The listing builds one solid part. Answer for the finished solid, in the listing's coordinates (mm). Face numbers are marked on the shaded views. A direction names the side the tool comes from. Round coordinates to 2 decimals unless told otherwise and drop trailing zeros. Order: outer loops, then holes, each group sorted by start corner. A loop starts at its lowest first (then second) coordinate and runs counter-clockwise, first axis right, second up. Notation, with made-up numbers: (66.25, 55) - (123.25, 55) arc R29 ccw to (123.25, 84) - close; hole circle Ø8 at (-2, 18.5). An arc over 180 degrees is marked (long way). Use CSV: the item, a comma, the result in double quotes. Start each with the question number.
Item 1: Find section D-D, the plane y = -2.1. Give the vertices of the cut face in (x, z), plus the area to 3 significant figures.
Item 2: For the marked faces 1 and 2, determine the directions among +Z, -Z, +X, -X, +Y, -Y from which every point of the face is accessible in a straight line to the end or side of a thin tool.
Item 3: Straight lines are drawn through the part: line 1 along Z through (x, y) = (-2.35, -1); line 2 along Z through (x, y) = (2.45, 0.4); line 3 along Y through (x, z) = (0, 1.5). For each, find the intervals that lie inside material, in ascending order. Write a range as [from, to].
Item 4: Flat-ended cylindrical pins translate along their axes: P1, Ø0.5, axis at x = 0, y = 0, coming from the +Z side; P2, Ø3, axis at x = 1, z = 23, coming from the +Y side; P3, Ø1.5, axis at x = -2, y = 0, coming from the -Z side; P4, Ø1.3, axis at x = -0.5, z = 26.5, coming from the -Y side. Find the tip coordinate at first contact, or state that the pin passes through.
Item 5: Find section A-A, the plane x = 0. Give the vertices of the cut face in (y, z).
Item 6: Find section C-C, the plane z = 18. Give the vertices of the cut face in (x, y).
Item 7: Find section B-B, the plane y = 0. Give the vertices of the cut face in (x, z).
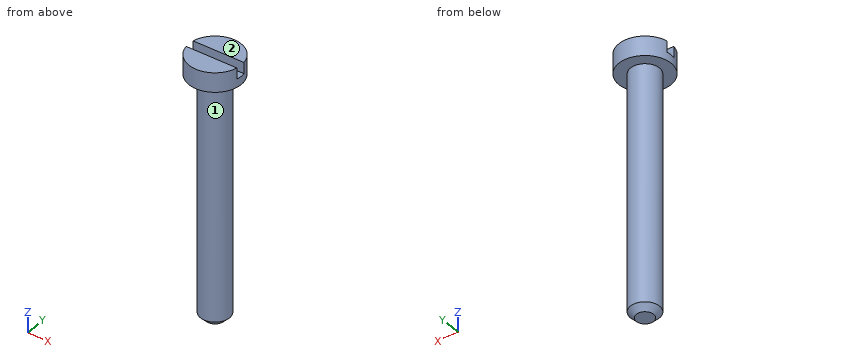
Solid Edge part; units mm, degrees
sketch "Sketch1" plane through (0, 0, 0) normal (0, 0, 1) x (1, 0, 0)
  circle A0 centre (0, 0) radius 1.5
extrude "Protrusion1" add sketch "Sketch1" along normal blind 25
chamfer "Chaflán_1" distance 0.6 angle 45 1 edges at (-1.5, 0, 0)
sketch "Sketch2" plane through (0, 0, 25) normal (0, 0, 1) x (1, 0, 0)
  circle A0 centre (0, 0) radius 2.7
extrude "ProtrusiónExtruida_3" add sketch "Sketch2" along normal blind 2
sketch "Sketch3" plane through (0, 0, 27) normal (0, 0, 1) x (0, 1, 0)
  line L0 (0.5, -3.2084) -> (-0.5, -3.2084)
  line L1 (-0.5, -3.2084) -> (-0.5, 3.2084)
  line L2 (-0.5, 3.2084) -> (0.5, 3.2084)
  line L3 (0.5, 3.2084) -> (0.5, -3.2084)
extrude "VaciadoExtruido_5" cut sketch "Sketch3" against normal blind 1.148
properties material "Acero inoxidable, 303"
Worked out:
1,outline,"(-1.7, 25) - (1.7, 25) - (1.7, 27) - (-1.7, 27) - close"
1,area,"6.79 mm²"
2,face 1,"-Z"
2,face 2,"+Z, +X, -X, +Y, -Y"
3,line 1,"z = [25, 27]"
3,line 2,"z = [25, 25.85]"
3,line 3,"y = [-1.5, 1.5]"
4,P1,"stops at z = 25.85"
4,P2,"stops at y = 1.5"
4,P3,"stops at z = 0.35"
4,P4,"stops at y = -2.7"
5,outline,"(-2.7, 25) - (-1.5, 25) - (-1.5, 0.6) - (-0.9, 0) - (0.9, 0) - (1.5, 0.6) - (1.5, 25) - (2.7, 25) - (2.7, 27) - (0.5, 27) - (0.5, 25.85) - (-0.5, 25.85) - (-0.5, 27) - (-2.7, 27) - close"
6,outline,"circle Ø3 at (0, 0)"
7,outline,"(-2.7, 25) - (-1.5, 25) - (-1.5, 0.6) - (-0.9, 0) - (0.9, 0) - (1.5, 0.6) - (1.5, 25) - (2.7, 25) - (2.7, 25.85) - (-2.7, 25.85) - close"
